For this review, take the finished solid that the model builds, in its own axes (mm). Coordinates: 2 decimals unless noted, no trailing zeros. Loops run counter-clockwise (first coordinate to the right, second up) from the corner with the lowest first, then second, coordinate; pieces in that order, holes last. Notation, with made-up numbers: M 37,14.5 L 85,14.5 A6 cw 85,19.5 Z; hole C 4,41 d4. An arc over 180 degrees is marked long. Put each result on its own line as item: value.
```python
from build123d import *

# Parameters (mm, degrees)
BOSS_EXTRU_1_START      = -10
BOSS_EXTRU_1_DEPTH      = 5
ESQUISSE2_R             = 3
ENL_V_MAT_EXTRU_1_DEPTH = 5


with BuildPart() as part:
    # Esquisse1 → Boss.-Extru.1 (new body)
    with BuildSketch(Plane.XY.offset(BOSS_EXTRU_1_START)):
        with BuildLine():
            Line((24.767075252, -5.790077162), (-46.257871267, -64.266200254))
            ThreePointArc((-46.257871267, -64.266200254), (-56.815023681, -63.243198344), (-55.792021772, -52.68604593))
            Line((-55.792021772, -52.68604593), (15.232924748, 5.790077162))
            ThreePointArc((15.232924748, 5.790077162), (25.790077162, 4.767075252), (24.767075252, -5.790077162))
        make_face()
    extrude(amount=BOSS_EXTRU_1_DEPTH)

    # Esquisse2 → Enlèv. mat.-Extru.1 (cut)
    with BuildSketch(Plane.XY.offset(-5)):
        with Locations((20, 0)):
            Circle(ESQUISSE2_R)
        with Locations((-51.024946519, -58.476123092)):
            Circle(ESQUISSE2_R)
    extrude(amount=-ENL_V_MAT_EXTRU_1_DEPTH, mode=Mode.SUBTRACT)


solid = part.part
```
(1) Add section A-A (y = 0). Write out the cut boundary in (x, z), plus the area to 3 significant figures.
Determined:
outline: M 8.2,-10 L 17,-10 L 17,-5 L 8.2,-5 Z; M 23,-10 L 27.5,-10 L 27.5,-5 L 23,-5 Z
area: 66.5 mm^2
(2) Draft analysis for pull direction Y (two halves, no side actions). For faces 1 (the cylindrical face through (25.684, 4.893, -7.535)), 2 (the cylindrical face through (-51.7, -61.4, -7.5)), 3 (the flat face through (-10.25, -34.62, -7.54)), state which applies: +Y half, -Y half, draft (parallel to the pull), parting line (faces both ways), or undercut.
Determined:
face 1: parting line
face 2: undercut
face 3: -Y half
(3) Add section B-B (x = 20). Write out the cut boundary in (y, z).
Determined:
outline: M -9.71,-10 L -3,-10 L -3,-5 L -9.71,-5 Z; M 3,-10 L 7.5,-10 L 7.5,-5 L 3,-5 Z
(4) For pin 1 (3 mm diameter, centred on y = -51, z = -7, fed in from +X); pin 2 (5 mm diameter, centred on x = 20, y = 0, fed in from +Z); pin 3 (3 mm diameter, centred on x = -18, z = -9, fed in from +Y); pin 4 (1.5 mm diameter, centred on x = -4.5, z = -8, fed in from -Y), all flat-tipped, find the tip position at first contact; note any pin that passes through.
Determined:
pin 1: stops at x = -28.32
pin 2: passes through
pin 3: stops at y = -20.34
pin 4: stops at y = -30.5
(5) Wall thickness on line 1 along Y through (x, z) = (20, -6); line 2 along Y through (x, z) = (-52, -7.7); line 3 along X through (y, z) = (-56, -5.8): over which ranges is each line inside the solid? List them lowest first. Write a range as [from, to].
Determined:
line 1: y = [-9.71, -3], [3, 7.5]
line 2: y = [-65.91, -61.31], [-55.64, -49.56]
line 3: x = [-58.1, -52.72], [-49.33, -36.22]
(6) Add section D-D (y = -17). Write out the cut boundary in (x, z), plus the area to 3 significant figures.
Determined:
outline: M -12.45,-10 L 11.15,-10 L 11.15,-5 L -12.45,-5 Z
area: 118 mm^2
(7) Add section C-C (z = -8.6). Write out the cut boundary in (x, y), plus the area to 3 significant figures.
Determined:
outline: M -55.79,-52.69 A7.5 ccw -46.26,-64.27 L 24.77,-5.79 A7.5 ccw 15.23,5.79 Z; hole C -51.02,-58.48 d6; hole C 20,0 d6
area: 1,500 mm^2
